The model under review builds one solid part; all positions refer to its coordinate system, in mm. Face numbers are marked on the shaded views. A direction names the side the tool comes from. Coordinates: 2 decimals unless noted, no trailing zeros. Order: outer loops, then holes, each group sorted by start corner. A loop starts at its lowest first (then second) coordinate and runs counter-clockwise, first axis right, second up. Notation, with made-up numbers: (-28.75, 86) -> (13.25, 86) arc R12 cw to (13.25, 108) -> close; hole circle Ø6 at (46.25, 58.25). An arc over 180 degrees is marked (long way). Put each result on its own line as item: value.
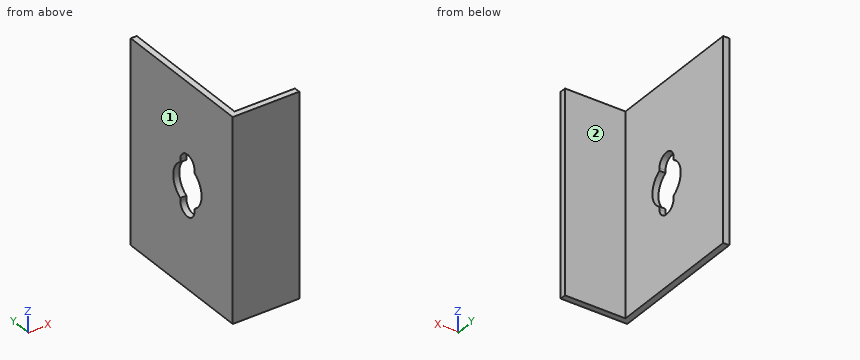
from build123d import *

# Parameters (mm, degrees)
BOSS_EXTRUDE1_DEPTH = 100
CUT_EXTRUDE1_DEPTH  = 100


with BuildPart() as part:
    # Sketch1 → Boss-Extrude1 (new body)
    with BuildSketch(Plane.XY):
        Polygon((0, 72), (3, 72), (3, 3), (33, 3), (33, 0), (0, 0), align=None)
    extrude(amount=BOSS_EXTRUDE1_DEPTH)

    # Sketch2 → Cut-Extrude1 (cut)
    with BuildSketch(Plane.ZY):
        with BuildLine():
            Line((58.660254038, 37), (60, 37))
            ThreePointArc((60, 37), (65, 32), (60, 27))
            Line((60, 27), (58.660254038, 27))
            ThreePointArc((58.660254038, 27), (50, 22), (41.339745962, 27))
            Line((41.339745962, 27), (40, 27))
            ThreePointArc((40, 27), (35, 32), (40, 37))
            Line((40, 37), (41.339745962, 37))
            ThreePointArc((41.339745962, 37), (50, 42), (58.660254038, 37))
        make_face()
    extrude(amount=-CUT_EXTRUDE1_DEPTH, mode=Mode.SUBTRACT)


solid = part.part
Item 1: For pin 1 Ø1.1 at (x, z) = (2, 59) entering from -Y; pin 2 Ø15 at (x, z) = (24, 52.5) entering from +Y; pin 3 Ø12 at (y, z) = (61, 62.5) entering from +X, all flat-tipped, find the tip position at first contact; note any pin that passes through.
Answers below:
pin 1: y = 0
pin 2: y = 3
pin 3: x = 3
Item 2: Consider section B-B on z = 43. Write out the cut boundary in (x, y), and give its area (3 significant figures).
Answers below:
outline: (0, 0) -> (33, 0) -> (33, 3) -> (3, 3) -> (3, 24.86) -> (0, 24.86) -> close; (0, 39.14) -> (3, 39.14) -> (3, 72) -> (0, 72) -> close
area: 263 mm^2
Item 3: For the marked faces 1 and 2, list the 3-axis set-ups (+Z, -Z, +X, -X, +Y, -Y) from which the entire face can be reached by the end or side of a thin tool; tool diameter is ignored.
Answers below:
face 1: +Z, -Z, -X, +Y, -Y
face 2: +Z, -Z, +X, +Y
Item 4: Consider section A-A on y = 32. Write out the cut boundary in (x, z), and give its area (3 significant figures).
Answers below:
outline: (0, 0) -> (3, 0) -> (3, 35) -> (0, 35) -> close; (0, 65) -> (3, 65) -> (3, 100) -> (0, 100) -> close
area: 210 mm^2
Item 5: Consider section D-D on x = 10.5. Write out the cut boundary in (y, z), and give its area (3 significant figures).
Answers below:
outline: (0, 0) -> (3, 0) -> (3, 100) -> (0, 100) -> close
area: 300 mm^2
Item 6: Consider section C-C on z = 75.5. Write out the cut boundary in (x, y), and give its area (3 significant figures).
Answers below:
outline: (0, 0) -> (33, 0) -> (33, 3) -> (3, 3) -> (3, 72) -> (0, 72) -> close
area: 306 mm^2
Item 7: For line 1 (Y direction, x = 18, z = 44.5), list the stretches that pass through material, from the lowest coordinate up. Write a range as from..to.
Answers below:
line 1: 0..3
